from build123d import *

# Parameters (mm, degrees)
SKETCH009_W     = 42
SKETCH009_H     = 55
SKETCH009_W_2   = 27
SKETCH009_H_2   = 40
PAD004_DEPTH    = 5
SKETCH010_R     = 2
POCKET004_DEPTH = 4
PAD005_DEPTH    = 20


with BuildPart() as part:
    # Sketch009 → Pad004 (new body)
    with BuildSketch(Plane.XY):
        Rectangle(SKETCH009_W, SKETCH009_H)
        Rectangle(SKETCH009_W_2, SKETCH009_H_2, mode=Mode.SUBTRACT)
    extrude(amount=PAD004_DEPTH)

    # Sketch010 → Pocket004 (cut)
    with BuildSketch(Plane.XY):
        with Locations((-17.25, 23.75)):
            Circle(SKETCH010_R)
        with Locations((17.25, 23.75)):
            Circle(SKETCH010_R)
        with Locations((17.25, -23.75)):
            Circle(SKETCH010_R)
        with Locations((-17.25, -23.75)):
            Circle(SKETCH010_R)
    extrude(amount=POCKET004_DEPTH, mode=Mode.SUBTRACT)

    # Sketch011 → Pad005 (join, symmetric)
    with BuildSketch(Plane(origin=(0, 0, 5), x_dir=(1, 0, 0), z_dir=(0, -1, 0))):
        Polygon((-13.5, 0), (-13.5, 5), (-12.8, 6.2), (-12.8, 6.6), (-13.5, 7), (-13.5, 7.8), (-12.9, 8.4), (-12.9, 8.8), (-13.5, 9.4), (-14.7, 9.4), (-16.5, 0), align=None)
    extrude(amount=PAD005_DEPTH, both=True)


with BuildPart() as part_1:
    # Body003 placement: moved
    add(part.part.moved(Location((-100, 0, 50))))


solid = part_1.part
Geometry: final body of the model. Coordinates: model frame, mm. A direction names the side the tool comes from. Round coordinates to 2 decimals unless told otherwise and drop trailing zeros. Loops run counter-clockwise (first coordinate to the right, second up) from the corner with the lowest first, then second, coordinate; pieces in that order, holes last. Notation, with made-up numbers: M 73,-31 L 95,-31 A22 ccw 95,4 Z; hole C 20,-3.75 d4. An arc over 180 degrees is marked long. One line per question, with ' | ' between items.
(1) Cut plane A-A on x = -90. Return the cut outline in (y, z), plus the area to 3 significant figures.
Check result:
outline: M -27.5,50 L -20,50 L -20,55 L -27.5,55 Z; M 20,50 L 27.5,50 L 27.5,55 L 20,55 Z | area: 75.0 mm2
(2) Cut plane D-D on x = -82.75. Return the cut outline in (y, z), plus the area to 3 significant figures.
Check result:
outline: M -27.5,50 L -25.75,50 L -25.75,54 L -21.75,54 L -21.75,50 L 21.75,50 L 21.75,54 L 25.75,54 L 25.75,50 L 27.5,50 L 27.5,55 L -27.5,55 Z | area: 243 mm2
(3) Pull-direction query (X, two-part tool) for faces 1 (the flat face through (-115, 20, 60)), 2 (the cylindrical face through (-80.842, 24.351, 51.972)), 3 (the flat face through (-79, 0, 52)); classes: +X half, -X half, draft (parallel to the pull), parting line (faces both ways), or undercut.
Check result:
face 1: draft | face 2: undercut | face 3: +X half
(4) Cut plane C-C on y = 23.75. Return the cut outline in (x, z), plus the area to 3 significant figures.
Check result:
outline: M -121,50 L -119.25,50 L -119.25,54 L -115.25,54 L -115.25,50 L -84.75,50 L -84.75,54 L -80.75,54 L -80.75,50 L -79,50 L -79,55 L -121,55 Z | area: 178 mm2
(5) Access query for faces 4 (the flat face through (-115, -20, 60)), 5 (the flat face through (-86.5, 0, 52)), 6 (the flat face through (-115.587, -0.28, 59.766)), 7 (the cylindrical face through (-119.248, 23.838, 51.972)), 8 (the flat face through (-100, 27.5, 52)). Directions: +Z, -Z, +X, -X, +Y, -Y. A direction counts if a zero-diameter tool reaches every point of the face in a straight line with its end or side. Return the directions, or none.
Check result:
face 4: +Z, +X, -X, -Y | face 5: +Z, -Z | face 6: +Z, -X, +Y, -Y | face 7: -Z | face 8: +Z, -Z, +X, -X, +Y
(6) Contact query for flat-ended pins moving along their axis: P1, Ø12, axis at x = -105.5, y = 8.5, coming from the -Z side; P2, Ø2, axis at x = -82.5, y = 24, coming from the -Z side; P3, Ø1.1, axis at x = -115, z = 59.5, coming from the +Y side; P4, Ø6.5, axis at x = -82.75, y = 23.75, coming from the -Z side. Output: stop coordinate, or through.
Check result:
P1: passes through | P2: stops at z = 54 | P3: stops at y = 20 | P4: stops at z = 50
(7) Cut plane B-B on y = -9.5. Return the cut outline in (x, z), plus the area to 3 significant figures.
Check result:
outline: M -121,50 L -113.5,50 L -113.5,60 L -112.8,61.2 L -112.8,61.6 L -113.5,62 L -113.5,62.8 L -112.9,63.4 L -112.9,63.8 L -113.5,64.4 L -114.7,64.4 L -116.5,55 L -121,55 Z; M -86.5,50 L -79,50 L -79,55 L -86.5,55 Z | area: 96.2 mm2
(8) Material intervals for line 1 along Y through (x, z) = (-117.25, 51.45); line 2 along Y through (x, z) = (-104, 52); line 3 along X through (y, z) = (0, 51.25), sorted ascending. Write a range as from..to.
Check result:
line 1: y = -27.5..-25.75, -21.75..21.75, 25.75..27.5 | line 2: y = -27.5..-20, 20..27.5 | line 3: x = -121..-113.5, -86.5..-79
